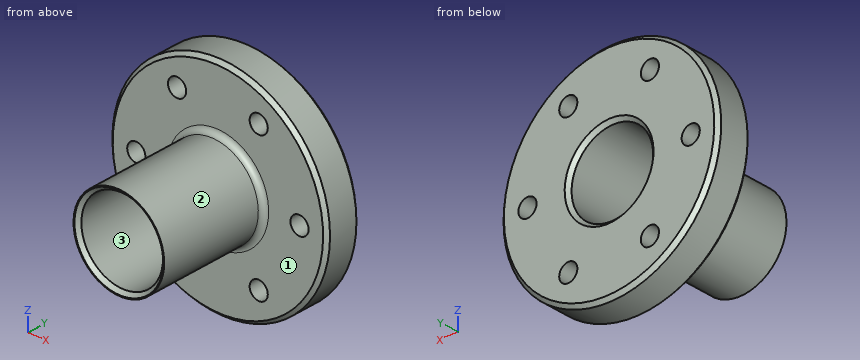
```python
from build123d import *

# Parameters (mm, degrees)
SKETCH2_R           = 60
SKETCH2_R_2         = 22.5
SKETCH2_R_3         = 5
BOSS_EXTRUDE1_DEPTH = 20
CHAMFER1_SIZE       = 2
CHAMFER2_SIZE       = 2
SKETCH3_R           = 25
BOSS_EXTRUDE2_DEPTH = 60
FILLET1_R           = 3
CUT_EXTRUDE1_START  = -60
SKETCH2_2_R         = 22.5
CUT_EXTRUDE1_DEPTH  = 60
CHAMFER3_SIZE       = 2
CHAMFER4_SIZE       = 2


with BuildPart() as part:
    # Sketch2 → Boss-Extrude1 (new body)
    with BuildSketch(Plane(origin=(0, 0, 0), x_dir=(1, 0, 0), z_dir=(0, 1, 0))):
        with Locations(Location((0, 0, 0), (0, 0, 270))):
            Circle(SKETCH2_R)
        with Locations(Location((0, 0, 0), (0, 0, 270))):
            Circle(SKETCH2_R_2, mode=Mode.SUBTRACT)
        with Locations(Location((45, 0, 0), (0, 0, 270))):
            Circle(SKETCH2_R_3, mode=Mode.SUBTRACT)
        with Locations(Location((22.5, -38.97114317, 0), (0, 0, 270))):
            Circle(SKETCH2_R_3, mode=Mode.SUBTRACT)
        with Locations(Location((-22.5, -38.97114317, 0), (0, 0, 270))):
            Circle(SKETCH2_R_3, mode=Mode.SUBTRACT)
        with Locations(Location((-45, 0, 0), (0, 0, 270))):
            Circle(SKETCH2_R_3, mode=Mode.SUBTRACT)
        with Locations(Location((-22.5, 38.97114317, 0), (0, 0, 270))):
            Circle(SKETCH2_R_3, mode=Mode.SUBTRACT)
        with Locations(Location((22.5, 38.97114317, 0), (0, 0, 270))):
            Circle(SKETCH2_R_3, mode=Mode.SUBTRACT)
    extrude(amount=BOSS_EXTRUDE1_DEPTH)

    # Chamfer1
    chamfer1_edges = [part.edges().sort_by_distance(p)[0] for p in [
        (0, 20, -60),
    ]]
    chamfer(chamfer1_edges, length=CHAMFER1_SIZE)

    # Chamfer2
    chamfer2_edges = [part.edges().sort_by_distance(p)[0] for p in [
        (0, 20, -22.5),
    ]]
    chamfer(chamfer2_edges, length=CHAMFER2_SIZE)

    # Sketch3 → Boss-Extrude2 (add)
    with BuildSketch(Plane(origin=(0, 0, 0), x_dir=(-1, 0, 0), z_dir=(0, -1, 0))):
        with Locations(Location((0, 0, 0), (0, 0, 270))):
            Circle(SKETCH3_R)
    extrude(amount=BOSS_EXTRUDE2_DEPTH)

    # Fillet1
    fillet1_edges = [part.edges().sort_by_distance(p)[0] for p in [
        (0, 0, -25),
    ]]
    fillet(fillet1_edges, radius=FILLET1_R)

    # Sketch2_2 → Cut-Extrude1 (cut)
    with BuildSketch(Plane(origin=(0, 0, 0), x_dir=(1, 0, 0), z_dir=(0, 1, 0)).offset(CUT_EXTRUDE1_START)):
        with Locations(Location((0, 0, 0), (0, 0, 270))):
            Circle(SKETCH2_2_R)
    extrude(amount=CUT_EXTRUDE1_DEPTH, mode=Mode.SUBTRACT)

    # Chamfer3
    chamfer3_edges = [part.edges().sort_by_distance(p)[0] for p in [
        (0, -60, -22.5),
    ]]
    chamfer(chamfer3_edges, length=CHAMFER3_SIZE)

    # Chamfer4
    chamfer4_edges = [part.edges().sort_by_distance(p)[0] for p in [
        (0, 0, -60),
    ]]
    chamfer(chamfer4_edges, length=CHAMFER4_SIZE)


solid = part.part
```
Geometry: final body of the model. Coordinates: model frame, mm. Face numbers are marked on the shaded views. Round coordinates to 2 decimals unless told otherwise and drop trailing zeros. Loops run counter-clockwise (first coordinate to the right, second up) from the corner with the lowest first, then second, coordinate; pieces in that order, holes last. Notation, with made-up numbers: (74, 1) -> (129, 1) arc R20 ccw to (129, 17) -> close; hole circle Ø7 at (32, 14). An arc over 180 degrees is marked (long way). Use one line per item in the form item = value.
Item 1: Draft query along Z for the marked faces 1, 2 and 3. Return one class per face: released by +Z, released by -Z, zero draft, split by the parting line, or undercut.
Evaluation:
face_1 = zero draft
face_2 = split by the parting line
face_3 = undercut
Item 2: Contact query for flat-ended pins moving along their axis: pin 1 Ø13 at (x, z) = (45, 0) entering from -Y; pin 2 Ø8 at (x, y) = (39, 0.5) entering from -Z; pin 3 Ø1 at (x, y) = (12, -8) entering from +Z. Output: stop coordinate, or through.
Evaluation:
pin_1 = 0
pin_2 = -48.52
pin_3 = 22.2
Item 3: Material intervals for probe 1 along X at (y, z) = (13.5, 0); probe 2 along X at (y, z) = (-50, 0.5) (3 decimals); probe 3 along X at (y, z) = (17, -38.5), sorted ascending.
Evaluation:
probe_1 = -60 to -50, -40 to -22.5, 22.5 to 40, 50 to 60
probe_2 = -24.995 to -22.494, 22.494 to 24.995
probe_3 = -46.02 to -27.48, -17.52 to 17.52, 27.48 to 46.02
Item 4: Cut plane D-D on y = -16.5. Output: boundary loops of the cut face in (x, z), then the cut area to 3 significant figures.
Evaluation:
outline = circle Ø50 at (0, 0); hole circle Ø45 at (0, 0)
area = 373 mm2
Item 5: Cut plane A-A on x = 0. Output: boundary loops of the cut face in (y, z).
Evaluation:
outline = (-60, -25) -> (-3, -25) arc R3 cw to (0, -28) -> (0, -58) -> (2, -60) -> (18, -60) -> (20, -58) -> (20, -24.5) -> (18, -22.5) -> (-58, -22.5) -> (-60, -24.5) -> close; (-60, 24.5) -> (-58, 22.5) -> (18, 22.5) -> (20, 24.5) -> (20, 58) -> (18, 60) -> (2, 60) -> (0, 58) -> (0, 28) arc R3 cw to (-3, 25) -> (-60, 25) -> close
Item 6: Cut plane B-B on z = 0. Give the number of separate pieces and of enclosed holes in the cut face, then the cut area to 3 significant figures.
Evaluation:
separate_pieces = 4
enclosed_holes = 0
area = 1,390 mm2
Item 7: Cut plane C-C on y = 7. Output: boundary loops of the cut face in (x, z), then the cut area to 3 significant figures.
Evaluation:
outline = circle Ø120 at (0, 0); hole circle Ø10 at (-45, 0); hole circle Ø10 at (-22.5, -38.97); hole circle Ø10 at (-22.5, 38.97); hole circle Ø45 at (0, 0); hole circle Ø10 at (22.5, -38.97); hole circle Ø10 at (22.5, 38.97); hole circle Ø10 at (45, 0)
area = 9,250 mm2
